from build123d import *

# Parameters (mm, degrees)
BOSS_EXTRUDE1_DEPTH = 3.175
SKETCH2_R           = 6.35
CUT_EXTRUDE1_DEPTH  = 4.175


with BuildPart() as part:
    # Sketch1 → Boss-Extrude1 (new body)
    with BuildSketch(Plane(origin=(0, 0, 0), x_dir=(1, 0, 0), z_dir=(0, 1, 0))):
        Polygon((-12.7, 6.35), (-12.7, 12.7), (12.7, 12.7), (12.7, 6.35), (15.875, 6.35), (15.875, -6.35), (12.7, -6.35), (12.7, -12.7), (-12.7, -12.7), (-12.7, -6.35), (-15.875, -6.35), (-15.875, 6.35), align=None)
    extrude(amount=BOSS_EXTRUDE1_DEPTH)

    # Sketch2 → Cut-Extrude1 (cut, through all)
    with BuildSketch(Plane(origin=(0, 3.175, 0), x_dir=(1, 0, 0), z_dir=(0, 1, 0))):
        Circle(SKETCH2_R)
    extrude(amount=-CUT_EXTRUDE1_DEPTH, mode=Mode.SUBTRACT)


solid = part.part
The listing builds one solid part. Answer for the finished solid, in the listing's coordinates (mm). A direction names the side the tool comes from. Round coordinates to 2 decimals unless told otherwise and drop trailing zeros. Order: outer loops, then holes, each group sorted by start corner. A loop starts at its lowest first (then second) coordinate and runs counter-clockwise, first axis right, second up. Notation, with made-up numbers: (-37.75, -24.5) -> (19.25, -24.5) arc R23 ccw to (19.25, -12.5) -> close; hole circle Ø5 at (-14, 5.25). An arc over 180 degrees is marked (long way). One line per item, written item: value.
Item 1: Straight lines are drawn through the part: L1, parallel to Z at x = 0, y = 2.55; L2, parallel to X at y = 2.5, z = 0 (3 decimals); L3, parallel to Z at x = 13.5, y = 2.95. For each, find the intervals that lie inside material, in ascending order.
Taken from the geometry:
L1: z = -12.7 to -6.35, 6.35 to 12.7
L2: x = -15.875 to -6.35, 6.35 to 15.875
L3: z = -6.35 to 6.35
Item 2: Find section B-B, the plane x = 0. Give the vertices of the cut face in (y, z) (3 decimals), then the cut area to 3 significant figures.
Taken from the geometry:
outline: (0, -12.7) -> (3.175, -12.7) -> (3.175, -6.35) -> (0, -6.35) -> close; (0, 6.35) -> (3.175, 6.35) -> (3.175, 12.7) -> (0, 12.7) -> close
area: 40.3 mm2
Item 3: For faces 1 (the flat face through (14, 2, -6.35)), 2 (the flat face through (-14, 2, -6.35)), 3 (the flat face through (-14, 2, 6.35)), determine the directions among +Z, -Z, +X, -X, +Y, -Y from which every point of the face is accessible in a straight line to the end or side of a thin tool.
Taken from the geometry:
face 1: -Z, +X, +Y, -Y
face 2: -Z, -X, +Y, -Y
face 3: +Z, -X, +Y, -Y
Item 4: Given P1, Ø1.6, axis at x = -14, y = 1, coming from the -Z side; P2, Ø1.6, axis at x = -14.5, y = 1, coming from the +Z side; P3, Ø1, axis at y = 2, z = -11, coming from the -X side, each flat-ended and moving along its own axis, determine where each tip first touches the part or whether it passes through.
Taken from the geometry:
P1: stops at z = -6.35
P2: stops at z = 6.35
P3: stops at x = -12.7
Item 5: Find section A-A, the plane z = 0. Give the vertices of the cut face in (x, y) (3 decimals), then the cut area to 3 significant figures.
Taken from the geometry:
outline: (-15.875, 0) -> (-6.35, 0) -> (-6.35, 3.175) -> (-15.875, 3.175) -> close; (6.35, 0) -> (15.875, 0) -> (15.875, 3.175) -> (6.35, 3.175) -> close
area: 60.5 mm2
Item 6: For a pull along X with two mould halves and no side action, classify faces 4 (the cylindrical face through (-1.38, 1.61, 6.2)), 5 (the flat face through (12.7, 2, 9)), 6 (the flat face through (-3, 3.175, -6)) as released by +X, released by -X, zero draft, split by the parting line, or undercut.
Taken from the geometry:
face 4: undercut
face 5: released by +X
face 6: zero draft
Item 7: Find section D-D, the plane z = -10.75. Give the vertices of the cut face in (x, y) (3 decimals), then the cut area to 3 significant figures.
Taken from the geometry:
outline: (-12.7, 0) -> (12.7, 0) -> (12.7, 3.175) -> (-12.7, 3.175) -> close
area: 80.6 mm2
Item 8: Find section C-C, the plane y = 1.25. Give the vertices of the cut face in (x, z) (3 decimals), then the cut area to 3 significant figures.
Taken from the geometry:
outline: (-15.875, -6.35) -> (-12.7, -6.35) -> (-12.7, -12.7) -> (12.7, -12.7) -> (12.7, -6.35) -> (15.875, -6.35) -> (15.875, 6.35) -> (12.7, 6.35) -> (12.7, 12.7) -> (-12.7, 12.7) -> (-12.7, 6.35) -> (-15.875, 6.35) -> close; hole circle Ø12.7 at (0, 0)
area: 599 mm2
